from build123d import *

# Parameters (mm, degrees)
F0_W     = 92
F0_H     = 60
F1_DEPTH = 0.3
F2_R     = 5
F3_R     = 1
F4_DEPTH = 0.7


with BuildPart() as f1:
    # F0 (on Top) → F1 (new body)
    with BuildSketch(Plane.XY):
        Rectangle(F0_W, F0_H)
    extrude(amount=F1_DEPTH)

    # F2
    f2_edges = [f1.edges().sort_by_distance(p)[0] for p in [
        (-46, 30, 0.15),
        (-46, -30, 0.15),
        (46, 30, 0.15),
        (46, -30, 0.15),
    ]]
    fillet(f2_edges, radius=F2_R)

    # F3 (on face) → F4 (join)
    with BuildSketch(Plane(origin=(0, 0, 0), x_dir=(1, 0, 0), z_dir=(0, 0, -1))):
        Circle(F3_R)
    extrude(amount=F4_DEPTH)


solid = f1.part
Geometry check sheet. Reference: the model listing, model coordinates, mm. A direction names the side the tool comes from. Give positions to 0.01 mm unless a question says otherwise; leave off trailing zeros. Loops run counter-clockwise (first coordinate to the right, second up) from the corner with the lowest first, then second, coordinate; pieces in that order, holes last. Notation, with made-up numbers: (74, 26) -> (104, 26) arc R21 cw to (104, 33) -> close; hole circle Ø9 at (63.5, 8). An arc over 180 degrees is marked (long way). Answer in a Markdown table with one row per item. Add a question column.
1) Cross-section at B-B on x = 0. Record the boundary of the cut face in (y, z).
2) Cross-section at C-C on z = -0.35. Record the boundary of the cut face in (x, y), and give its area (3 significant figures).
3) Cross-section at D-D on x = -20. Record the boundary of the cut face in (y, z).
4) Cross-section at A-A on y = 0. Record the boundary of the cut face in (x, z).
5) Set-up check for faces 1 (the face through (-0.217, 0.976, -0.345)), 2 (the face through (0, 0, -0.7)): record each of +Z, -Z, +X, -X, +Y, -Y from which the full face is reachable in a straight line by a thin tool's end or side.
6) Material ranges on probe 1 along Z at (x, y) = (0, -23.5), recorded low to high. Write a range as from..to.
Outcome:
| question | item | result |
|---|---|---|
| 1 | outline | (-30, 0) -> (-1, 0) -> (-1, -0.7) -> (1, -0.7) -> (1, 0) -> (30, 0) -> (30, 0.3) -> (-30, 0.3) -> close |
| 2 | outline | circle Ø2 at (0, 0) |
| 2 | area | 3.14 mm^2 |
| 3 | outline | (-30, 0) -> (30, 0) -> (30, 0.3) -> (-30, 0.3) -> close |
| 4 | outline | (-46, 0) -> (-1, 0) -> (-1, -0.7) -> (1, -0.7) -> (1, 0) -> (46, 0) -> (46, 0.3) -> (-46, 0.3) -> close |
| 5 | face 1 | -Z |
| 5 | face 2 | -Z, +X, -X, +Y, -Y |
| 6 | probe 1 | z = 0..0.3 |
